Part model, mm, in its own coordinate system. A direction names the side the tool comes from. Coordinates: 2 decimals unless noted, no trailing zeros. Write each loop counter-clockwise with the first axis right and the second up, starting at its lowest first coordinate (ties: lowest second). Pieces come first, ordered by that corner, then holes. Notation, with made-up numbers: (9.5, -26) - (37.5, -26) arc R20 cw to (37.5, -19) - close; hole circle Ø9 at (56.25, -10). An arc over 180 degrees is marked (long way). Write each question's results on one line, items separated by ' | '.
from build123d import *

# Parameters (mm, degrees)
F1_DEPTH  = 25
F3_DEPTH  = 60
F4_R      = 15.3734931233
F5_DEPTH  = 131.1684809697
F8_DEPTH  = 6
F10_DEPTH = 6
F11_R     = 25
F12_R     = 25
F14_D     = 5.1054
F14_DEPTH = 25
F14_TIP   = 1.5338169022
F15_D     = 6.7564
F15_DEPTH = 25
F15_TIP   = 2.0298273432
F16_D     = 4.1
F16_DEPTH = 25
F16_TIP   = 1.231764269
F18_DEPTH = 5


with BuildPart() as f1:
    # F0 (on Top) → F1 (new body)
    with BuildSketch(Plane.XY):
        with BuildLine():
            ThreePointArc((45, 0), (0, -45), (-45, 0))
            Line((-45, 0), (-68, 0))
            Line((-68, 0), (-68, -4.880737979))
            Line((-68, -4.880737979), (-52.2726352577, -4.880737979))
            ThreePointArc((-52.2726352577, -4.880737979), (-31.783629524, -41.7857738265), (9.2519405818, -51.678347453))
            Line((9.2519405818, -51.678347453), (37.5362118293, -79.9626187004))
            Line((37.5362118293, -79.9626187004), (79.9626187004, -37.5362118293))
            Line((79.9626187004, -37.5362118293), (68, -25.5735931288))
            Line((68, -25.5735931288), (68, 0))
            Line((68, 0), (45, 0))
        make_face()
    extrude(amount=F1_DEPTH)

    # F2 (on face) → F3 (join)
    with BuildSketch(Plane(origin=(0, 0, 0), x_dir=(1, 0, 0), z_dir=(0, 0, -1))):
        Polygon((79.9626187004, 37.5362118293), (37.5362118293, 79.9626187004), (33.2935711421, 75.7199780133), (75.7199780133, 33.2935711421), align=None)
    extrude(amount=F3_DEPTH)

    # F4 (on face) → F5 (cut, through all)
    with BuildSketch(Plane(origin=(58.7494152648, -58.7494152648, 0), x_dir=(0.7071067812, 0.7071067812, 0), z_dir=(0.7071067812, -0.7071067812, 0))):
        with Locations((0, -30)):
            Circle(F4_R)
    extrude(amount=-F5_DEPTH, mode=Mode.SUBTRACT)

    # F7 (on face) → F8 (join)
    with BuildSketch(Plane(origin=(-21.2132034356, -21.2132034356, 0), x_dir=(0.7071067812, -0.7071067812, 0), z_dir=(-0.7071067812, -0.7071067812, 0))):
        Polygon((83.084219849, -60), (83.084219849, 25), (36.7878936231, 25), (36.7878936231, 0), (77.084219849, -60), align=None)
    extrude(amount=F8_DEPTH)

    # F9 (on face) → F10 (join)
    with BuildSketch(Plane(origin=(21.2132034356, 21.2132034356, 0), x_dir=(-0.7071067812, 0.7071067812, 0), z_dir=(0.7071067812, 0.7071067812, 0))):
        Polygon((-83.084219849, 25), (-83.084219849, -60), (-77.084219849, -60), (-36.1771658063, 0), (-36.1771658063, 25), align=None)
    extrude(amount=F10_DEPTH)

    # F11
    f11_edges = [f1.edges().sort_by_distance(p)[0] for p in [
        (1.564981, -52.476669, 12.5),
    ]]
    fillet(f11_edges, radius=F11_R)

    # F12
    f12_edges = [f1.edges().sort_by_distance(p)[0] for p in [
        (68, -17.088312, 12.5),
    ]]
    fillet(f12_edges, radius=F12_R)

    # F14
    with Locations(Plane(origin=(0, 0, 0), x_dir=(-1, 0, 0), z_dir=(0, 1, 0))):
        with Locations((-60, 6), (-60, 19)):
            Hole(F14_D / 2, depth=F14_DEPTH)
            with Locations((0, 0, -(F14_DEPTH + F14_TIP / 2))):  # 118° drill point
                Cone(0, F14_D / 2, F14_TIP, mode=Mode.SUBTRACT)

    # F15
    with Locations(Plane(origin=(0, 0, 0), x_dir=(-1, 0, 0), z_dir=(0, 1, 0))):
        with Locations((60, 6), (60, 19)):
            Hole(F15_D / 2, depth=F15_DEPTH)
            with Locations((0, 0, -(F15_DEPTH + F15_TIP / 2))):  # 118° drill point
                Cone(0, F15_D / 2, F15_TIP, mode=Mode.SUBTRACT)

    # F16
    with Locations(Plane(origin=(58.7494152648, -58.7494152648, 0), x_dir=(0.7071067812, 0.7071067812, 0), z_dir=(0.7071067812, -0.7071067812, 0))):
        with Locations((-24, -6), (24, -6), (24, -54), (-24, -54)):
            Hole(F16_D / 2, depth=F16_DEPTH)
            with Locations((0, 0, -(F16_DEPTH + F16_TIP / 2))):  # 118° drill point
                Cone(0, F16_D / 2, F16_TIP, mode=Mode.SUBTRACT)

    # F17 (on face) → F18 (join)
    with BuildSketch(Plane.XY.offset(25)):
        Polygon((72.0430227512, -45.4558077785), (79.114090563, -52.5268755904), (80.5283041254, -51.112662028), (73.4572363135, -44.0415942162), align=None)
        Polygon((51.112662028, -80.5283041254), (52.5268755904, -79.114090563), (45.4558077785, -72.0430227512), (44.0415942162, -73.4572363135), align=None)
    extrude(amount=-F18_DEPTH)


solid = f1.part
(1) 3-axis set-ups, long thin cutter, end or side, ignore diameter. For faces 1 (the cylindrical face through (57.45, -12.67, 19.11)), 2 (the flat face through (49.04, -75.63, 22.54)), 3 (the flat face through (49, -76, 20)), 4 (the flat face through (75.22, -24.31, -16.9)): which of +Z, -Z, +X, -X, +Y, -Y reach the whole face in a straight line?
Return value:
face 1: +Y | face 2: +Z, -Z, +X | face 3: -Z, +X, -Y | face 4: -Z, +X, +Y
(2) Flat gauge pins, fed straight in: P1, Ø6.5, axis at x = 60, z = 19, coming from the -Y side; P2, Ø11, axis at x = -60, z = 19, coming from the -Y side; P3, Ø5, axis at y = -27.5, z = -17.5, coming from the -X side; P4, Ø9, axis at x = -60, z = 6, coming from the +Y side. Where does each tip first touch, or does it go through?
Return value:
P1: stops at y = -60.75 | P2: stops at y = -4.88 | P3: stops at x = 67.43 | P4: stops at y = 0
(3) Saw through at A-A on x = -60. Write the cut outline in (y, z), then the cut area to 3 significant figures.
Return value:
outline: (-4.88, 0) - (0, 0) - (0, 2.62) - (-4.88, 2.62) - close; (-4.88, 9.38) - (0, 9.38) - (0, 15.62) - (-4.88, 15.62) - close; (-4.88, 22.38) - (0, 22.38) - (0, 25) - (-4.88, 25) - close | area: 56.1 mm^2
(4) Wall check: line 1 (Z direction, x = 60, y = -18); line 2 (Z direction, x = 45.5, y = -27); line 3 (Z direction, x = 60, y = -16.25). Give the ranges that are in metal, low to high. Write a range as from..to.
Return value:
line 1: z = 0..3.45, 8.55..16.45, 21.55..25 | line 2: z = 0..25 | line 3: z = -26.02..3.45, 8.55..16.45, 21.55..25
(5) Saw through at B-B on z = -19. Write the cut outline in (x, y), then the cut area to 3 significant figures.
Return value:
outline: (9.58, -60.49) - (33.29, -84.21) - (51.16, -66.34) - (46.91, -62.1) - (33.29, -75.72) - (13.82, -56.25) - close; (55.95, -13.53) - (75.72, -33.29) - (62.1, -46.91) - (66.34, -51.16) - (84.21, -33.29) - (60.2, -9.29) - close | area: 636 mm^2
(6) Two-plate mould, pull along Z, no slides. Class faces 5 (the cylindrical face through (57.45, -12.67, 6.11)), 6 (the flat face through (77, -48, 20)), 7 (the flat face through (44.782, -64.232, -16.247)): released by +Z, released by -Z, zero draft, split by the parting line, or undercut.
Return value:
face 5: undercut | face 6: released by -Z | face 7: zero draft
